Design review of the part built by this model. Coordinates are the model's own, in mm. A direction names the side the tool comes from. Coordinates: 2 decimals unless noted, no trailing zeros. Write each loop counter-clockwise with the first axis right and the second up, starting at its lowest first coordinate (ties: lowest second). Pieces come first, ordered by that corner, then holes. Notation, with made-up numbers: (-28.75, 53) - (29.25, 53) arc R29 ccw to (29.25, 90) - close; hole circle Ø6 at (4.25, -36.75). An arc over 180 degrees is marked (long way). Use a Markdown table: item, result.
from build123d import *

# Parameters (mm, degrees)
F0_W     = 76.2
F0_H     = 76.2
F0_R     = 7.62
F0_R_2   = 5.08
F1_DEPTH = 6.35
F2_DEPTH = 132.08
F3_DEPTH = 5.08


# Not quite as in the source:
# - a feature names something its author has since deleted; it is built from what else it names


with BuildPart() as f1:
    # F0 (on Top) → F1 (new body)
    with BuildSketch(Plane.XY):
        with Locations((-17.4512108788, -34.2747404939)):
            Rectangle(F0_W, F0_H)
        with Locations((-46.3251647948, -5.4007865778)):
            Circle(F0_R, mode=Mode.SUBTRACT)
        with Locations((-46.3251647948, -5.4007865778)):
            Circle(F0_R)
        with Locations((-46.3251647948, -5.4007865778)):
            Circle(F0_R_2, mode=Mode.SUBTRACT)
        with Locations((-46.3251647948, -5.4007865778)):
            Circle(F0_R_2)
    extrude(amount=-F1_DEPTH)

    # F0 (on Top) → F2 (join)
    with BuildSketch(Plane.XY):
        with Locations((-46.3251647948, -5.4007865778)):
            Circle(F0_R_2)
    extrude(amount=F2_DEPTH)

    # F0 (on Top) → F3 (join)
    with BuildSketch(Plane.XY):
        with Locations((-46.3251647948, -5.4007865778)):
            Circle(F0_R)
        with Locations((-46.3251647948, -5.4007865778)):
            Circle(F0_R_2, mode=Mode.SUBTRACT)
    extrude(amount=F3_DEPTH)


solid = f1.part
(1) Take a section at C-C on z = 86.5. Write out the cut boundary in (x, y), and give its area (3 significant figures).
Determined:
| item | result |
|---|---|
| outline | circle Ø10.16 at (-46.33, -5.4) |
| area | 81.1 mm2 |
(2) For L1, parallel to Z at x = -34.5, y = -36; L2, parallel to X at y = -2.5, z = 42; L3, parallel to X at y = -9, z = 43.5, list the stretches that pass through material, from the lowest coordinate up. Write a range as from..to.
Determined:
| item | result |
|---|---|
| L1 | -6.35..0 |
| L2 | -50.5..-42.15 |
| L3 | -49.91..-42.74 |
(3) Take a section at B-B on y = -8.5. Write out the cut boundary in (x, z).
Determined:
| item | result |
|---|---|
| outline | (-55.55, -6.35) - (20.65, -6.35) - (20.65, 0) - (-39.36, 0) - (-39.36, 5.08) - (-42.3, 5.08) - (-42.3, 132.08) - (-50.35, 132.08) - (-50.35, 5.08) - (-53.29, 5.08) - (-53.29, 0) - (-55.55, 0) - close |
(4) For pin 1 (5 mm diameter, centred on x = -48, z = 28.5, fed in from +Y); pin 2 (4 mm diameter, centred on x = -30.5, y = -4, fed in from +Z); pin 3 (1 mm diameter, centred on x = -43, z = 43.5, fed in from -Y), all flat-tipped, find the tip position at first contact; note any pin that passes through.
Determined:
| item | result |
|---|---|
| pin 1 | y = -0.32 |
| pin 2 | z = 0 |
| pin 3 | y = -9.62 |
(5) Take a section at A-A on x = -49. Write out the cut boundary in (y, z), and give its area (3 significant figures).
Determined:
| item | result |
|---|---|
| outline | (-72.37, -6.35) - (3.83, -6.35) - (3.83, 0) - (1.73, 0) - (1.73, 5.08) - (-1.08, 5.08) - (-1.08, 132.08) - (-9.72, 132.08) - (-9.72, 5.08) - (-12.54, 5.08) - (-12.54, 0) - (-72.37, 0) - close |
| area | 1,650 mm2 |
(6) Machinability: for faces 1 (the flat face through (-41, -7, 5.08)), 2 (the flat face through (-18, 3.825, -3)), which of the approach directions +Z, -Z, +X, -X, +Y, -Y give a long, thin tool a straight path to every point of the face, cutting with its end or side? Answer none if there is none.
Determined:
| item | result |
|---|---|
| face 1 | +Z |
| face 2 | +Z, -Z, +X, -X, +Y |
(7) Take a section at D-D on y = -44. Write out the cut boundary in (x, z).
Determined:
| item | result |
|---|---|
| outline | (-55.55, -6.35) - (20.65, -6.35) - (20.65, 0) - (-55.55, 0) - close |
